Autodesk Inventor part; units mm, degrees
ref_plane "YZ Plane" through (0, 0, 0) normal (1, 0, 0) x (0, 1, 0)
ref_plane "XZ Plane" through (0, 0, 0) normal (0, 1, 0) x (-1, 0, 0)
ref_plane "XY Plane" through (0, 0, 0) normal (0, 0, 1) x (1, 0, 0)
sketch "Sketch1" plane through (0, 0, 0) normal (0, 0, 1) x (1, 0, 0)
  line L0 (0, 0) -> (38.1, 0)
  line L1 (38.1, 0) -> (38.1, -26.9875)
  line L2 (0, 0) -> (0, -26.9875)
  line L3 (0, -26.9875) -> (7.5012, -43.3836)
  line L4 (38.1, -26.9875) -> (30.5988, -43.3836)
  arc A0 (7.5012, -43.3836) -> (30.5988, -43.3836) centre (19.05, -38.1) ccw
  line L5 (38.1, -25.4) -> (0, -25.4) construction
  line L6 (38.1, -26.9875) -> (0, -26.9875) construction
  line L7 (38.1, -23.8125) -> (0, -23.8125) construction
  dimension "d1" = 38.1
  dimension "d2" = 12.7
  dimension "d36" = 38.1
  dimension "d37" = 25.4
  dimension "d38" = 1.5875
  dimension "d39" = 1.5875
extrude "Extrusion1" add sketch "Sketch1" along normal blind 3.175
sketch "Sketch2" plane through (0, 0, 0) normal (0, 0, -1) x (-1, 0, 0)
  line L0 (-38.1, 0) -> (-38.1, -26.9875)
  line L1 (0, -26.9875) -> (0, 0)
  line L2 (-38.1, -26.9875) -> (0, -26.9875)
  line L3 (0, -26.9875) -> (0, -23.8125)
  line L4 (0, -23.8125) -> (-38.1, -23.8125)
  line L5 (-38.1, -23.8125) -> (-38.1, -26.9875)
  arc A0 (-7.5012, -43.3836) -> (-30.5988, -43.3836) centre (-19.05, -38.1) ccw
  dimension "d13" = 3.175
extrude "Extrusion2" add sketch "Sketch2" along normal blind 34.925
sketch "Sketch3" plane through (0, 0, 3.175) normal (0, 0, 1) x (1, 0, 0)
  line L0 (7.5012, -43.3836) -> (0, -26.9875)
  arc A0 (30.5988, -43.3836) -> (7.5012, -43.3836) centre (19.05, -38.1) ccw
  line L1 (0, -26.9875) -> (0, 0)
  line L2 (0, 0) -> (38.1, 0)
  line L3 (38.1, 0) -> (38.1, -26.9875)
  line L4 (38.1, -23.8125) -> (0, -23.8125)
  line L5 (38.1, -23.8125) -> (0, -23.8125)
  point P0 (9.525, -14.2875)
  point P1 (28.575, -6.35)
  dimension "d18" = 9.525
  dimension "d20" = 6.35
  dimension "d21" = 9.525
  dimension "d40" = 9.525
hole "Hole1" at (9.525, -14.2875, 3.175) at (28.575, -6.35, 3.175) direction (0, 0, -1) diameter 5.1054 end through all
sketch "Sketch4" plane through (0, 0, 3.175) normal (0, 0, 1) x (1, 0, 0)
  arc A0 (30.5988, -43.3836) -> (7.5012, -43.3836) centre (19.05, -38.1) ccw
  point P0 (0, 0)
hole "Hole2" at (19.05, -38.1, 3.175) direction (0, 0, -1) diameter 6.35 end through all
properties part number "CLB_087_ClimberMountBracketGusset" material "Aluminum 6061"
Input: part model. Units: mm. Frame: model coordinates. A direction names the side the tool comes from. Coordinates: 2 decimals unless noted, no trailing zeros. Write each loop counter-clockwise with the first axis right and the second up, starting at its lowest first coordinate (ties: lowest second). Pieces come first, ordered by that corner, then holes. Notation, with made-up numbers: (18.5, -13.75) -> (24.5, -13.75) arc R25 ccw to (24.5, 17.25) -> close; hole circle Ø9 at (33.5, 19). An arc over 180 degrees is marked (long way). Answer as a JSON object with one key per item and string values.
1. Section C-C on z = -17. Return the cut outline in (x, y).
Result set:
{"outline": "(0, -26.99) -> (38.1, -26.99) -> (38.1, -23.81) -> (0, -23.81) -> close"}
2. First-contact query: P1, Ø2, axis at x = 11, z = -20, coming from the -Y side; P2, Ø19, axis at x = 25, y = -44, coming from the -Z side; P3, Ø3, axis at x = 27.5, z = -4, coming from the +Y side. Flat tips, straight axial feed; report the tip coordinate or a pass-through.
Result set:
{"P1": "stops at y = -26.99", "P2": "stops at z = 0", "P3": "stops at y = -23.81"}
3. Section B-B on x = 27. Return the cut outline in (y, z) (1 decimal).
Result set:
{"outline": "(-48, 0) -> (-27, 0) -> (-27, -34.9) -> (-23.8, -34.9) -> (-23.8, 0) -> (-8.4, 0) -> (-8.4, 3.2) -> (-48, 3.2) -> close; (-4.3, 0) -> (0, 0) -> (0, 3.2) -> (-4.3, 3.2) -> close"}
4. Section D-D on x = 15. Return the cut outline in (y, z) (1 decimal), then the cut area to 3 significant figures.
Result set:
{"outline": "(-50.1, 0) -> (-27, 0) -> (-27, -34.9) -> (-23.8, -34.9) -> (-23.8, 0) -> (0, 0) -> (0, 3.2) -> (-50.1, 3.2) -> close", "area": "270 mm2"}
5. Access query for faces 1 (the face through (11.078, -12.262, 1.565)), 2 (the face through (19, -33, 0)), 3 (the face through (19, -12, 0)). Directions: +Z, -Z, +X, -X, +Y, -Y. A direction counts if a zero-diameter tool reaches every point of the face in a straight line with its end or side. Return the directions, or none.
Result set:
{"face 1": "+Z, -Z", "face 2": "-Z, +X, -X, -Y", "face 3": "-Z, +X, -X, +Y"}
6. Mould query, pull axis X, two halves, no side actions, for faces 4 (the face through (18.91, -34.93, 1.57)), 5 (the face through (31.067, -5.797, 1.565)), 6 (the face through (19, 0, 2)), 7 (the face through (0, -24, -9)). Classes: released by +X, released by -X, zero draft, split by the parting line, or undercut.
Result set:
{"face 4": "undercut", "face 5": "undercut", "face 6": "zero draft", "face 7": "released by -X"}
7. Section A-A on y = -6.35. Return the cut outline in (x, z) (3 decimals), then the cut area to 3 significant figures.
Result set:
{"outline": "(0, 0) -> (26.022, 0) -> (26.022, 3.175) -> (0, 3.175) -> close; (31.128, 0) -> (38.1, 0) -> (38.1, 3.175) -> (31.128, 3.175) -> close", "area": "105 mm2"}
8. Material intervals for line 1 (Y direction, x = 19.05, z = 1) (3 decimals); line 2 (Z direction, x = 34, y = -16) (3 decimals); line 3 (Y direction, x = 14, z = -8), sorted ascending. Write a range as from..to.
Result set:
{"line 1": "y = -50.8..-41.275, -34.925..0", "line 2": "z = 0..3.175", "line 3": "y = -26.99..-23.81"}
